Source: CAD feature listing. Evaluate the final solid. Frame: model axes, mm. Face numbers are marked on the shaded views. A direction names the side the tool comes from. Round coordinates to 2 decimals unless told otherwise and drop trailing zeros. Write each loop counter-clockwise with the first axis right and the second up, starting at its lowest first coordinate (ties: lowest second). Pieces come first, ordered by that corner, then holes.
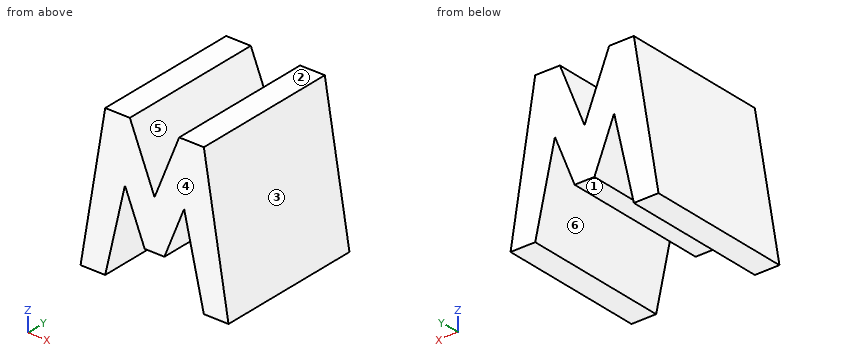
```python
from build123d import *

# Parameters (mm, degrees)
F2_DEPTH = 38.1


with BuildPart() as f2:
    # F1 (on offset) → F2 (new body)
    with BuildSketch(Plane.XZ.offset(38.1)):
        Polygon((6.35, 38.1), (0, 0), (6.35, 0), (11.43, 22.225), (16.51, 9.525), (21.59, 9.525), (26.67, 22.225), (31.75, 0), (38.1, 0), (31.75, 38.1), (25.4, 38.1), (19.05, 22.225), (12.7, 38.1), align=None)
    extrude(amount=F2_DEPTH)


solid = f2.part
```
Q1. Section query A-A, the plane y = -40.5. Output: boundary loops of the cut face in (x, z) (3 decimals), and give its area (3 significant figures).
Q2. Pin query (flat end, axial travel): P1, Ø3, axis at y = -43, z = 32.5, coming from the +X side; P2, Ø5, axis at y = -50, z = 18.5, coming from the +X side; P3, Ø3, axis at y = -60, z = 22, coming from the +X side. Return the tip coordinate at first contact, or that it passes through.
Q3. Section query C-C, the plane z = 16.5. Output: boundary loops of the cut face in (x, y), and give its area (3 significant figures).
Q4. Section query D-D, the plane x = 15.5. Output: boundary loops of the cut face in (y, z), and give its area (3 significant figures).
Q5. Section query B-B, the plane z = 8.5. Output: boundary loops of the cut face in (x, y), and give its area (3 significant figures).
Q6. Line query: line 1 (X direction, y = -60.5, z = 10); line 2 (X direction, y = -62, z = 20); line 3 (X direction, y = -56, z = 24.5). Output: solid intervals per line, ascending.
Q7. Mould query, pull axis X, two halves, no side actions, for the marked faces 1, 2 and 3. Classes: pulls with the +X half, pulls with the -X half, needs draft (parallel to the pull), parting line crosses it, or undercut.
Q8. Set-up query: the marked faces 4, 5 and 6. Return all of +Z, -Z, +X, -X, +Y, -Y with unobstructed straight access to the full face (end or side cutting, diameter ignored); none if empty.
Filled in:
1. outline: (0, 0) - (6.35, 0) - (11.43, 22.225) - (16.51, 9.525) - (21.59, 9.525) - (26.67, 22.225) - (31.75, 0) - (38.1, 0) - (31.75, 38.1) - (25.4, 38.1) - (19.05, 22.225) - (12.7, 38.1) - (6.35, 38.1) - close
1. area: 786 mm2
2. P1: stops at x = 32.93
2. P2: stops at x = 35.43
2. P3: stops at x = 34.68
3. outline: (2.75, -76.2) - (10.12, -76.2) - (10.12, -38.1) - (2.75, -38.1) - close; (13.72, -76.2) - (24.38, -76.2) - (24.38, -38.1) - (13.72, -38.1) - close; (27.98, -76.2) - (35.35, -76.2) - (35.35, -38.1) - (27.98, -38.1) - close
3. area: 968 mm2
4. outline: (-76.2, 12.05) - (-38.1, 12.05) - (-38.1, 31.1) - (-76.2, 31.1) - close
4. area: 726 mm2
5. outline: (1.42, -76.2) - (8.29, -76.2) - (8.29, -38.1) - (1.42, -38.1) - close; (29.81, -76.2) - (36.68, -76.2) - (36.68, -38.1) - (29.81, -38.1) - close
5. area: 524 mm2
6. line 1: x = 1.67 to 8.64, 16.32 to 21.78, 29.46 to 36.43
6. line 2: x = 3.33 to 10.92, 12.32 to 25.78, 27.18 to 34.77
6. line 3: x = 4.08 to 18.14, 19.96 to 34.02
7. face 1: undercut
7. face 2: needs draft
7. face 3: pulls with the +X half
8. face 4: +Z, -Z, +X, -X, -Y
8. face 5: +Z, +Y, -Y
8. face 6: -Z, +Y, -Y
